```python
from build123d import *

# Parameters (mm, degrees)
F0_R     = 21
F1_DEPTH = 100
F4_R     = 20
F4_R_2   = 17
F5_DEPTH = 25


with BuildPart() as f1:
    # F0 (on Top) → F1 (new body)
    with BuildSketch(Plane.XY):
        Circle(F0_R)
    extrude(amount=F1_DEPTH)

    # F2 (on Front) → F3 (revolve)
    with BuildSketch(Plane.XZ):
        Polygon((-24, 85), (0, 85), (0, 141), (-24, 141), (-29, 136), (-29, 118), (-24, 113), align=None)
    revolve(axis=Axis((0, 0, 74.559175), (0, 0, 1)))

    # F4 (on face) → F5 (join)
    with BuildSketch(Plane.XY.offset(141)):
        Circle(F4_R)
        Circle(F4_R_2, mode=Mode.SUBTRACT)
    extrude(amount=F5_DEPTH)


solid = f1.part
```
Design review of the part built by this model. Coordinates are the model's own, in mm. A direction names the side the tool comes from. Coordinates: 2 decimals unless noted, no trailing zeros. Order: outer loops, then holes, each group sorted by start corner. A loop starts at its lowest first (then second) coordinate and runs counter-clockwise, first axis right, second up. Notation, with made-up numbers: M 33,8.5 L 90,8.5 A26 cw 90,47.5 Z; hole C 55,3 d9. An arc over 180 degrees is marked long. Answer as a JSON object with one key per item and string values. Group by question number.
1) Add section C-C, the plane z = 65.5. Write out the cut boundary in (x, y), then the cut area to 3 significant figures.
2) Tool access review of faces 1 (the flat face through (-9, -15, 166)), 2 (the flat face through (0, 0, 141)), 3 (the flat face through (0.1, 21.2, 85)): name each direction out of +Z, -Z, +X, -X, +Y, -Y from which nothing blocks a thin tool from reaching the whole face with its end or side.
3) Mouldability with a two-part tool opening along Y and no side actions: class faces 4 (the conical face through (-23.19, -7.3, 140.69)), 5 (the flat face through (0, 0, 0)), 6 (the cylindrical face through (9.139, 14.334, 153.325)) as pulls with the +Y half, pulls with the -Y half, needs draft (parallel to the pull), parting line crosses it, or undercut.
4) Add section D-D, the plane z = 103. Write out the cut boundary in (x, y), then the cut area to 3 significant figures.
5) Add section A-A, the plane y = 0. Write out the cut boundary in (x, z).
6) Wall thickness on L1, parallel to Y at x = 0, z = 158; L2, parallel to Z at x = 1, y = -14; L3, parallel to Z at x = 2, y = 21: over which ranges is each line inside the solid? List them lowest first.
7) For pin 1 (1.5 mm diameter, centred on x = -13.5, y = 14, fed in from -Z); pin 2 (3 mm diameter, centred on y = -20, z = 20.5, fed in from -X); pin 3 (12 mm diameter, centred on x = -13, z = 82, fed in from +Y); pin 4 (4 mm diameter, centred on y = -10.5, z = 58, fed in from +X), all flat-tipped, find the tip position at first contact; note any pin that passes through.
Computed values:
{
 "1": {"outline": "C 0,0 d42", "area": "1,390 mm^2"},
 "2": {"face 1": "+Z, +X, -X, +Y, -Y", "face 2": "+Z", "face 3": "-Z"},
 "3": {"face 4": "parting line crosses it", "face 5": "needs draft", "face 6": "undercut"},
 "4": {"outline": "C 0,0 d48", "area": "1,810 mm^2"},
 "5": {"outline": "M -29,118 L -24,113 L -24,85 L -21,85 L -21,0 L 21,0 L 21,85 L 24,85 L 24,113 L 29,118 L 29,136 L 24,141 L 20,141 L 20,166 L 17,166 L 17,141 L -17,141 L -17,166 L -20,166 L -20,141 L -24,141 L -29,136 Z"},
 "6": {"L1": "y = -20 to -17, 17 to 20", "L2": "z = 0 to 141", "L3": "z = 85 to 141"},
 "7": {"pin 1": "stops at z = 0", "pin 2": "stops at x = -9.94", "pin 3": "stops at y = 22.7", "pin 4": "stops at x = 19.2"}
}
